```python
from build123d import *

# Parameters (mm, degrees)
CHAMFER1_SIZE  = 0.25
CHAMFER2_SIZE  = 0.5
CHAMFER3_SIZE  = 3
CHAMFER3_SIZE2 = 4.28444402


with BuildPart() as part:
    # Sketch2 → Revolve1 (revolve)
    with BuildSketch(Plane(origin=(0, 0, 0), x_dir=(1, 0, 0), z_dir=(0, 1, 0)), mode=Mode.PRIVATE) as revolve1_sk:
        Polygon((44.8, 14), (44.8, 0), (49, 0), (49, 12), (46.8, 12), (46.8, 14), align=None)
    revolve(revolve1_sk.sketch.rotate(Axis((0, 0, -51.275510204), (0, 0, 1)), 180), axis=Axis((0, 0, -51.275510204), (0, 0, 1)))

    # Chamfer1
    chamfer1_edges = [part.edges().sort_by_distance(p)[0] for p in [
        (46.8, 0, -14),
    ]]
    chamfer(chamfer1_edges, length=CHAMFER1_SIZE)

    # Chamfer2
    chamfer2_edges = [part.edges().sort_by_distance(p)[0] for p in [
        (49, 0, -12),
    ]]
    chamfer(chamfer2_edges, length=CHAMFER2_SIZE)

    # Chamfer3
    chamfer3_edges = [part.edges().sort_by_distance(p)[0] for p in [
        (49, 0, 0),
    ]]
    chamfer3_side = [part.faces().sort_by_distance(p)[0] for p in [
        (46.185929291, 0, 0),
    ]]
    chamfer(chamfer3_edges, length=CHAMFER3_SIZE, length2=CHAMFER3_SIZE2, reference=chamfer3_side[0])


solid = part.part
```
Check sheet for the modelled part. Datum: model origin and axes. Units: mm. A direction names the side the tool comes from. Round coordinates to 2 decimals unless told otherwise and drop trailing zeros. Order: outer loops, then holes, each group sorted by start corner. A loop starts at its lowest first (then second) coordinate and runs counter-clockwise, first axis right, second up. Notation, with made-up numbers: (1.5, 6.25) -> (22.5, 6.25) arc R31 ccw to (22.5, 36.25) -> close; hole circle Ø5 at (61.5, 7). An arc over 180 degrees is marked (long way). One line per item, written item: value. Start each with the question number.
Q1. Cross-section at A-A (x = 0). Record the boundary of the cut face in (y, z).
Q2. Set-up check for faces 4 (the face through (-21.595, 41.52, -12.887)), 5 (the face through (10.01, 45.09, -0.27)): record each of +Z, -Z, +X, -X, +Y, -Y from which the full face is reachable in a straight line by a thin tool's end or side.
Q3. Cross-section at C-C (z = -6.5). Record the boundary of the cut face in (x, y).
Q4. Gauge pin test, flat ends, axial feed: pin 1 Ø6 at (x, z) = (6, -7.5) entering from -Y; pin 2 Ø1.5 at (x, z) = (39, -3.5) entering from -Y; pin 3 Ø5 at (x, z) = (-21.5, -11) entering from +Y; pin 4 Ø5 at (x, y) = (32.5, -32) entering from +Z. Record the tip position at first contact, or that the pin passes through.
Q5. Mould release check, pull along X, two halves, no side actions. Record for faces 1 (the face through (44.757, -1.97, -6.902)), 2 (the face through (10, 44, 0)), 3 (the face through (-26.34, -41.32, -7.94)): pulls with the +X half, pulls with the -X half, needs draft (parallel to the pull), parting line crosses it, or undercut.
Q6. Thickness scan on line 1 (Y direction, x = 0, z = -9); line 2 (X direction, y = -12.5, z = -7.5); line 3 (Y direction, x = 14, z = -0.5). Record the ranges inside material, lowest first.
Completed:
1. outline: (-49, -11.5) -> (-48.5, -12) -> (-46.8, -12) -> (-46.8, -13.75) -> (-46.55, -14) -> (-44.8, -14) -> (-44.8, 0) -> (-46, 0) -> (-49, -4.28) -> close; (44.8, -14) -> (46.55, -14) -> (46.8, -13.75) -> (46.8, -12) -> (48.5, -12) -> (49, -11.5) -> (49, -4.28) -> (46, 0) -> (44.8, 0) -> close
2. face 4: -Z
2. face 5: +Z
3. outline: circle Ø98 at (0, 0); hole circle Ø89.6 at (0, 0)
4. pin 1: stops at y = -48.91
4. pin 2: stops at y = -30.06
4. pin 3: stops at y = 45.17
4. pin 4: stops at z = 0
5. face 1: undercut
5. face 2: needs draft
5. face 3: parting line crosses it
6. line 1: y = -49 to -44.8, 44.8 to 49
6. line 2: x = -47.38 to -43.02, 43.02 to 47.38
6. line 3: y = -44.19 to -42.56, 42.56 to 44.19
